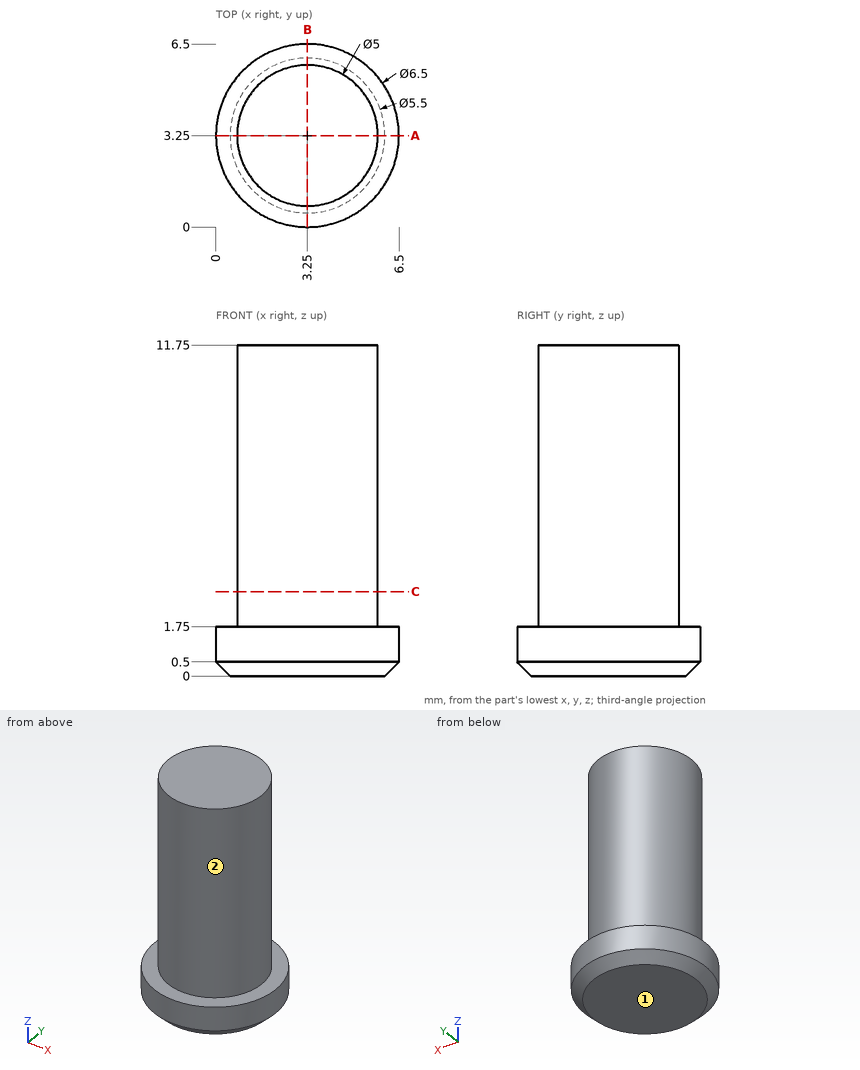
Study the drawing (mm; zero at the part's minimum x, y, z) and answer. A direction names the side the tool comes from. Give positions to 0.01 mm unless a question says otherwise; leave off trailing zeros. Order: outer loops, then holes, each group sorted by start corner. A loop starts at its lowest first (then second) coordinate and runs counter-clockwise, first axis right, second up. Notation, with made-up numbers: (61.25, 38.25) -> (112.25, 38.25) arc R18 ccw to (112.25, 69.25) -> close; hole circle Ø10 at (81, 55.5). An arc over 180 degrees is marked (long way). Write item = value, one per line.
1. A cutting plane is placed at C-C, the plane z = 3. Write down the section's boundary in (x, y).
Numbers:
outline = circle Ø5 at (3.25, 3.25)
2. Given pin 1 (2 mm diameter, centred on y = 4.5, z = 2, fed in from -X); pin 2 (2 mm diameter, centred on x = 2, z = 9.5, fed in from -Y); pin 3 (3 mm diameter, centred on x = 1, z = 5.5, fed in from +Y), each flat-ended and moving along its own axis, determine where each tip first touches the part or whether it passes through.
Numbers:
pin_1 = 0.01
pin_2 = 0.76
pin_3 = 5.63
3. For the marked faces 1 and 2, determine the directions among +Z, -Z, +X, -X, +Y, -Y from which every point of the face is accessible in a straight line to the end or side of a thin tool.
Numbers:
face_1 = -Z, +X, -X, +Y, -Y
face_2 = +Z
4. A cutting plane is placed at A-A, the plane y = 3.25. Write down the section's boundary in (x, z).
Numbers:
outline = (0, 0.5) -> (0.5, 0) -> (6, 0) -> (6.5, 0.5) -> (6.5, 1.75) -> (5.75, 1.75) -> (5.75, 11.75) -> (0.75, 11.75) -> (0.75, 1.75) -> (0, 1.75) -> close
5. Straight lines are drawn through the part: line 1 along Z through (x, y) = (3, 6.25); line 2 along Y through (x, z) = (2.5, 2); line 3 along Y through (x, z) = (5.25, 9.5). For each, find the intervals that lie inside material, in ascending order.
Numbers:
line_1 = 0.26 to 1.75
line_2 = 0.87 to 5.63
line_3 = 1.75 to 4.75
